from build123d import *

# Parameters (mm, degrees)
CROQUIS1_W              = 19
CROQUIS1_H              = 5
CROQUIS1_R              = 1.6
SALIENTE_EXTRUIR1_DEPTH = 4.2
CROQUIS2_R              = 4.009695102
CORTAR_EXTRUIR1_DEPTH   = 7.2


with BuildPart() as part:
    # Croquis1 → Saliente-Extruir1 (new body)
    with BuildSketch(Plane.XY):
        with Locations((25.783027827, -30.609692022)):
            Rectangle(CROQUIS1_W, CROQUIS1_H)
        with Locations((19.34510909, -30.609692022)):
            Circle(CROQUIS1_R, mode=Mode.SUBTRACT)
        with Locations((32.220946564, -30.609692022)):
            Circle(CROQUIS1_R, mode=Mode.SUBTRACT)
    extrude(amount=SALIENTE_EXTRUIR1_DEPTH)

    # Croquis2 → Cortar-Extruir1 (cut)
    with BuildSketch(Plane.XZ.offset(33.109692022)):
        with Locations((25.783027827, -2.383165564)):
            Circle(CROQUIS2_R)
    extrude(amount=-CORTAR_EXTRUIR1_DEPTH, mode=Mode.SUBTRACT)


solid = part.part
Read the model definition and answer for the solid it produces. Units are mm, in the model's axes. Coordinates: 2 decimals unless noted, no trailing zeros. Order: outer loops, then holes, each group sorted by start corner. A loop starts at its lowest first (then second) coordinate and runs counter-clockwise, first axis right, second up. Notation, with made-up numbers: (0.5, -7) - (10.5, -7) arc R13 cw to (10.5, 10) - close; hole circle Ø6 at (65.5, -21.5). An arc over 180 degrees is marked (long way). Use one line per item in the form item = value.
(1) Section D-D, the plane y = -28.65 is taken. Give the vertices of the cut face in (x, z), then the cut area to 3 significant figures.
Computed values:
outline = (16.28, 0) - (22.56, 0) arc R4.01 cw to (29.01, 0) - (35.28, 0) - (35.28, 4.2) - (16.28, 4.2) - close
area = 72.5 mm²
(2) Section A-A, the plane z = 1.35 is taken. Give the vertices of the cut face in (x, y).
Computed values:
outline = (16.28, -33.11) - (24.32, -33.11) - (24.32, -28.11) - (16.28, -28.11) - close; (27.25, -33.11) - (35.28, -33.11) - (35.28, -28.11) - (27.25, -28.11) - close; hole circle Ø3.2 at (19.35, -30.61); hole circle Ø3.2 at (32.22, -30.61)
(3) Straight lines are drawn through the part: L1, parallel to X at y = -30.7, z = 2.8; L2, parallel to X at y = -31.2, z = 1.3; L3, parallel to X at y = -29.7, z = 0.5. For each, find the intervals that lie inside material, in ascending order.
Computed values:
L1 = 16.28 to 17.75, 20.94 to 30.62, 33.82 to 35.28
L2 = 16.28 to 17.86, 20.83 to 24.2, 27.37 to 30.73, 33.71 to 35.28
L3 = 16.28 to 18.03, 20.66 to 23, 28.57 to 30.9, 33.54 to 35.28
(4) For a pull along X with two mould halves and no side action, classify faces 1 (the face through (16.283, -31, 2)), 2 (the face through (31, -29, 0)), 3 (the face through (25.835, -30.645, 1.626)) as pulls with the +X half, pulls with the -X half, needs draft (parallel to the pull), parting line crosses it, or undercut.
Computed values:
face_1 = pulls with the -X half
face_2 = needs draft
face_3 = undercut
(5) Section C-C, the plane x = 33 is taken. Give the vertices of the cut face in (y, z), then the cut area to 3 significant figures.
Computed values:
outline = (-33.11, 0) - (-32.01, 0) - (-32.01, 4.2) - (-33.11, 4.2) - close; (-29.21, 0) - (-28.11, 0) - (-28.11, 4.2) - (-29.21, 4.2) - close
area = 9.26 mm²
(6) Section B-B, the plane y = -31.2 is taken. Give the vertices of the cut face in (x, z).
Computed values:
outline = (16.28, 0) - (17.86, 0) - (17.86, 4.2) - (16.28, 4.2) - close; (20.83, 0) - (22.56, 0) arc R4.01 cw to (29.01, 0) - (30.73, 0) - (30.73, 4.2) - (20.83, 4.2) - close; (33.71, 0) - (35.28, 0) - (35.28, 4.2) - (33.71, 4.2) - close
